```python
from build123d import *

# Parameters (mm, degrees)
EXTRUDE_1_DEPTH          = 5
EXTRUDE_2_DEPTH          = 5
PATTERN_CIRCULAR_1_COUNT = 4
SKETCH_3_R               = 10
EXTRUDE_3_DEPTH          = 5
PATTERN_CIRCULAR_2_COUNT = 4
SKETCH_4_R               = 0.8
CUT_EXTRUDE_1_DEPTH      = 219


with BuildPart() as part:
    # 草图1 → 凸台-拉伸1 (new, symmetric)
    with BuildSketch(Plane.XY):
        Polygon((-20, 10), (20, 10), (20, 0), (5, 0), (5, -80), (20, -80), (20, -90), (-20, -90), (-20, -80), (-5, -80), (-5, 0), (-20, 0), align=None)
    extrude(amount=EXTRUDE_1_DEPTH, both=True)

    # 草图2 → 凸台-拉伸2 (add)
    with BuildSketch(Plane.XZ.offset(90)):
        Polygon((65.40737726, 61.871843354), (61.871843354, 65.40737726), (-1.767766953, 1.767766953), (1.767766953, -1.767766953), align=None)
    extrude_2 = extrude(amount=-EXTRUDE_2_DEPTH)

    # 阵列(圆周)1: 凸台-拉伸2 ×4 about axis
    pattern_circular_1_axis = Axis((0, 0, 0), (0, 1, 0))
    for i in range(1, PATTERN_CIRCULAR_1_COUNT):
        add(extrude_2.rotate(pattern_circular_1_axis, i * 360 / PATTERN_CIRCULAR_1_COUNT))

    # 草图3 → 凸台-拉伸3 (add)
    with BuildSketch(Plane(origin=(0, -85, 0), x_dir=(1, 0, 0), z_dir=(0, 1, 0))):
        with Locations((63.639610307, 63.639610307)):
            Circle(SKETCH_3_R)
    extrude_3 = extrude(amount=-EXTRUDE_3_DEPTH)

    # 阵列(圆周)2: 凸台-拉伸3 ×4 about axis
    pattern_circular_2_axis = Axis((0, 0, 0), (0, 1, 0))
    for i in range(1, PATTERN_CIRCULAR_2_COUNT):
        add(extrude_3.rotate(pattern_circular_2_axis, i * 360 / PATTERN_CIRCULAR_2_COUNT))

    # 草图4 → 切除-拉伸1 (cut)
    with BuildSketch(Plane(origin=(0, 10, 0), x_dir=(1, 0, 0), z_dir=(0, 1, 0))):
        with Locations(Location((15, 0, 0), (0, 0, 180))):
            Circle(SKETCH_4_R)
        with Locations(Location((-15, 0, 0), (0, 0, 270))):
            Circle(SKETCH_4_R)
    extrude(amount=-CUT_EXTRUDE_1_DEPTH, mode=Mode.SUBTRACT)


solid = part.part
```
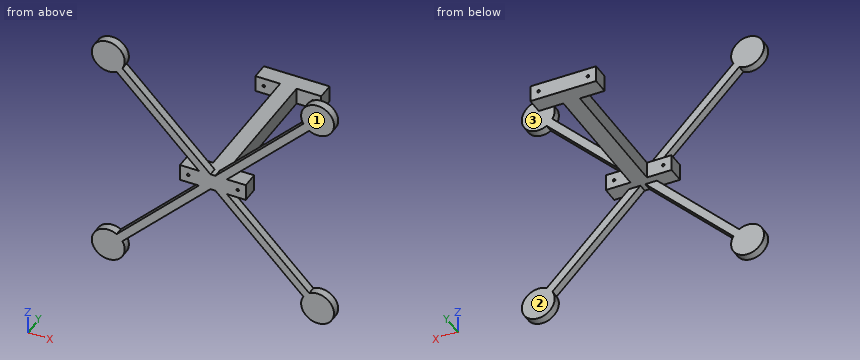
Could you check a few things on this model? Use its own coordinates, in mm. Face numbers are marked on the shaded views. A direction names the side the tool comes from. Round coordinates to 2 decimals unless told otherwise and drop trailing zeros. Loops run counter-clockwise (first coordinate to the right, second up) from the corner with the lowest first, then second, coordinate; pieces in that order, holes last. Notation, with made-up numbers: (88, 15.25) -> (107, 15.25) arc R30 ccw to (107, 51.25) -> close; hole circle Ø11 at (84.5, 40). An arc over 180 degrees is marked (long way). Put each result on its own line as item: value.
Q1. I want a section at B-B on x = -29.5. Write out the boundary of the cut face in (y, z).
Checks:
outline: (-90, -33.04) -> (-85, -33.04) -> (-85, -25.96) -> (-90, -25.96) -> close; (-90, 25.96) -> (-85, 25.96) -> (-85, 33.04) -> (-90, 33.04) -> close
Q2. Which directions (+Z, -Z, +X, -X, +Y, -Y) give clear straight access to the entire face, cutting with the end or side of a thin tool? Please do the marked faces 1, 2 and 3.
Checks:
face 1: +Z, -Z, +X, -X, -Y
face 2: -Z, +X, -X, +Y
face 3: +Z, +X, -X, +Y
Q3. I want a section at A-A on z = -22.5. Write out the boundary of the cut face in (x, y).
Checks:
outline: (-26.04, -90) -> (-18.96, -90) -> (-18.96, -85) -> (-26.04, -85) -> close; (18.96, -90) -> (26.04, -90) -> (26.04, -85) -> (18.96, -85) -> close
Q4. I want a section at C-C on y = -31.5. Write out the boundary of the cut face in (x, z), and give its area (3 significant figures).
Checks:
outline: (-5, -5) -> (5, -5) -> (5, 5) -> (-5, 5) -> close
area: 100 mm2
Q5. Please list where these lines run through material, in increasing order: line 1 (Z direction, x = 15, y = 7.75); line 2 (Z direction, x = 15, y = -86); line 3 (Z direction, x = 1, y = -81). Write a range as from..to.
Checks:
line 1: -5..-0.8, 0.8..5
line 2: -18.54..-11.46, -5..-0.8, 0.8..5, 11.46..18.54
line 3: -5..5
Q6. For pin 1 Ø20 at (x, y) = (-4.5, -30.5) entering from -Z; pin 2 Ø3 at (x, y) = (1.5, -32) entering from +Z; pin 3 Ø5 at (y, z) = (3.5, -0.5) entering from -X, each with a flat end and sliding along its axis, tell me the tip position at first contact or that it passes through.
Checks:
pin 1: z = -5
pin 2: z = 5
pin 3: x = -20
